Autodesk Inventor part; units mm, degrees
ref_plane "XZ Plane" through (0, 0, 0) normal (0, 1, 0) x (-1, 0, 0)
ref_plane "XY Plane" through (0, 0, 0) normal (0, 0, 1) x (1, 0, 0)
sketch "Sketch1" plane through (0, 0, 0) normal (0, 0, 1) x (1, 0, 0)
  line L0 (0, 0) -> (200, 0) construction
  line L1 (200, 0) -> (200, 22) construction
  line L2 (200, 22) -> (0, 22) construction
  line L3 (0, 22) -> (0, 0) construction
  line L4 (200, 22) -> (145, 22) construction
  line L5 (145, 22) -> (145, 0) construction
  line L6 (145, 0) -> (200, 0) construction
  line L7 (200, 0) -> (200, 22) construction
  line L8 (200, 11) -> (0, 11) construction
  arc A0 (5, 16) -> (5, 6) centre (5, 11) ccw
  circle A1 centre (10, 11) radius 2
  circle A2 centre (19, 11) radius 2
  arc A3 (195, 6) -> (195, 16) centre (195, 11) ccw
  circle A4 centre (145, 11) radius 8 construction
  circle A5 centre (145, 19) radius 1.5
  circle A6 centre (137, 11) radius 1.5
  circle A7 centre (145, 11) radius 8 construction
  circle A8 centre (145, 3) radius 1.5
  circle A9 centre (153, 11) radius 1.5
  line L9 (132.51, 16) -> (5, 16)
  line L10 (195, 16) -> (157.49, 16)
  line L11 (195, 6) -> (157.49, 6)
  line L12 (132.51, 6) -> (5, 6)
  arc A10 (136.4131, 4.125) -> (153.5869, 4.125) centre (145, 11) ccw
  arc A11 (153.5869, 17.875) -> (136.4131, 17.875) centre (145, 11) ccw
  circle A12 centre (195, 11) radius 2
  circle A13 centre (177, 11) radius 2
  arc A14 (132.51, 16) -> (136.4131, 17.875) centre (132.51, 21) ccw
  arc A15 (136.4131, 4.125) -> (132.51, 6) centre (132.51, 1) ccw
  arc A16 (153.5869, 17.875) -> (157.49, 16) centre (157.49, 21) ccw
  arc A17 (157.49, 6) -> (153.5869, 4.125) centre (157.49, 1) ccw
  point P0 (135.202, 16)
  point P1 (154.798, 6)
  point P2 (135.202, 6)
  point P3 (154.798, 16)
  dimension "d0" = 200
  dimension "d1" = 22
  dimension "d2" = 55
  dimension "d7" = 4
  dimension "d8" = 4
  dimension "d9" = 9
  dimension "d10" = 10
  dimension "d11" = 16
  dimension "d12" = 3
  dimension "d13" = 3
  dimension "d14" = 4
  dimension "d15" = 4
  dimension "d16" = 18
  dimension "d17" = 5
extrude "Extrusion1" add sketch "Sketch1" along normal blind 3.7
sketch "Sketch2" plane through (0, 0, 0) normal (1, 0, 0) x (0, 1, 0)
  point P0 (0, 0)
ref_plane "Work Plane1" through (0, 0, 0) normal (1, 0, 0) x (0, 1, 0)
properties part number "Pendulo" material "PMMA Plastic"
The listing builds one solid part. Answer for the finished solid, in the listing's coordinates (mm). A direction names the side the tool comes from. Coordinates: 2 decimals unless noted, no trailing zeros. Loops run counter-clockwise (first coordinate to the right, second up) from the corner with the lowest first, then second, coordinate; pieces in that order, holes last. Notation, with made-up numbers: M -28.75,70 L -7.75,70 A14 ccw -7.75,80 Z; hole C 49,38.5 d8. An arc over 180 degrees is marked long. Answer as a JSON object with one key per item and string values. Group by question number.
Item 1: Section B-B (z = 1.1) is taken. Give the number of separate pieces and of enclosed holes in the cut face, and give its area (3 significant figures).
Item 2: Section A-A (x = 19) is taken. Write down the section's boundary in (y, z), and give its area (3 significant figures).
Item 3: Which of the six approach directions +Z, -Z, +X, -X, +Y, -Y give full straight-line access (tool end or side, diameter ignored) to faces 1 (the face through (177, 16, 2)), 2 (the face through (177, 6, 2)), 3 (the face through (70, 16, 2)), 4 (the face through (70, 6, 2)), 5 (the face through (10, 9, 2))?
Item 4: Determine the mould class of faces 6 (the face through (99, 11, 3.7)), 7 (the face through (134.65, 5.52, 1.82)), 8 (the face through (193, 11, 2)) for opening direction X: +X half, -X half, draft (parallel to the pull), parting line (faces both ways), or undercut.
Item 5: Each of these flat-tipped pins is pushed along its axis until it touches: P1, Ø1.1, axis at x = 183, z = 2, coming from the -Y side; P2, Ø1, axis at y = 7.5, z = 1.5, coming from the +X side; P3, Ø1.1, axis at x = 67.5, z = 1, coming from the +Y side. Where does it stop, or does it pass through?
Item 6: Section C-C (x = 63.5) is taken. Write down the section's boundary in (y, z).
Item 7: Consider L1, parallel to X at y = 9.25, z = 1.2; L2, parallel to Y at x = 19, z = 2.35; L3, parallel to Y at x = 42.5, z = 3.15. Determine where each line is inside the solid, lowest interval first.
Solved:
{
 "1": {"separate pieces": "1", "enclosed holes": "8", "area": "2,070 mm2"},
 "2": {"outline": "M 6,0 L 9,0 L 9,3.7 L 6,3.7 Z; M 13,0 L 16,0 L 16,3.7 L 13,3.7 Z", "area": "22.2 mm2"},
 "3": {"face 1": "+Z, -Z, +X, +Y", "face 2": "+Z, -Z, +X, -Y", "face 3": "+Z, -Z, -X, +Y", "face 4": "+Z, -Z, -X, -Y", "face 5": "+Z, -Z"},
 "4": {"face 6": "draft", "face 7": "-X half", "face 8": "undercut"},
 "5": {"P1": "stops at y = 6", "P2": "stops at x = 199", "P3": "stops at y = 16"},
 "6": {"outline": "M 6,0 L 16,0 L 16,3.7 L 6,3.7 Z"},
 "7": {"L1": "x = 0.32 to 9.03, 10.97 to 18.03, 19.97 to 176.03, 177.97 to 194.03, 195.97 to 199.68", "L2": "y = 6 to 9, 13 to 16", "L3": "y = 6 to 16"}
}
